CAD build for the part. Positions are in the model's coordinates, mm. Round coordinates to 2 decimals unless told otherwise and drop trailing zeros. Loops run counter-clockwise (first coordinate to the right, second up) from the corner with the lowest first, then second, coordinate; pieces in that order, holes last. Notation, with made-up numbers: M 39.5,-2.75 L 80.5,-2.75 A19 ccw 80.5,11.25 Z; hole C -31.5,-16 d2. An arc over 180 degrees is marked long. Use one line per item in the form item = value.
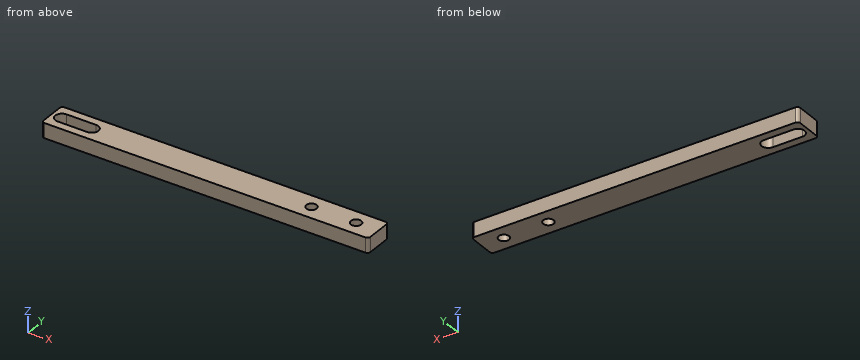
from build123d import *

# Parameters (mm, degrees)
F0_R     = 3.5
F1_DEPTH = 10


with BuildPart() as f1:
    # F0 (on Top) → F1 (new body)
    with BuildSketch(Plane.XY):
        with BuildLine():
            ThreePointArc((0, 2), (0.585786, 0.585786), (2, 0))
            Line((2, 0), (218, 0))
            ThreePointArc((218, 0), (219.414214, 0.585786), (220, 2))
            Line((220, 2), (220, 18))
            ThreePointArc((220, 18), (219.414214, 19.414214), (218, 20))
            Line((218, 20), (2, 20))
            ThreePointArc((2, 20), (0.585786, 19.414214), (0, 18))
            Line((0, 18), (0, 2))
        make_face()
        with BuildLine():
            ThreePointArc((7, 5.5), (2.5, 10), (7, 14.5))
            Line((7, 14.5), (27, 14.5))
            ThreePointArc((27, 14.5), (31.5, 10), (27, 5.5))
            Line((27, 5.5), (7, 5.5))
        make_face(mode=Mode.SUBTRACT)
        with Locations((175, 10)):
            Circle(F0_R, mode=Mode.SUBTRACT)
        with Locations((205, 10)):
            Circle(F0_R, mode=Mode.SUBTRACT)
    extrude(amount=F1_DEPTH)


solid = f1.part
1. Cut at C-C on x = 17. Write the cut outline in (y, z), and give its area (3 significant figures).
Completed:
outline = M 0,0 L 5.5,0 L 5.5,10 L 0,10 Z; M 14.5,0 L 20,0 L 20,10 L 14.5,10 Z
area = 110 mm2
2. Cut at B-B on z = 3.75. Write the cut outline in (x, y).
Completed:
outline = M 0,2 A2 ccw 2,0 L 218,0 A2 ccw 220,2 L 220,18 A2 ccw 218,20 L 2,20 A2 ccw 0,18 Z; hole M 7,5.5 L 27,5.5 A4.5 ccw 27,14.5 L 7,14.5 A4.5 ccw Z; hole C 175,10 d7; hole C 205,10 d7
3. Probe line 1 along X through (y, z) = (9.75, 9.25); line 2 along Y through (x, z) = (23.5, 3); line 3 along Y through (x, z) = (205, 5.25). List the from-to ranges inside material, lowest first. Write a range as from..to.
Completed:
line_1 = 0..2.51, 31.49..171.51, 178.49..201.51, 208.49..220
line_2 = 0..5.5, 14.5..20
line_3 = 0..6.5, 13.5..20
4. Cut at A-A on x = 175. Write the cut outline in (y, z), and give its area (3 significant figures).
Completed:
outline = M 0,0 L 6.5,0 L 6.5,10 L 0,10 Z; M 13.5,0 L 20,0 L 20,10 L 13.5,10 Z
area = 130 mm2
